Drawing for the job (mm, zero at the part's lowest x, y, z). A direction names the side the tool comes from. Give positions to 0.01 mm unless a question says otherwise; leave off trailing zeros. Order: outer loops, then holes, each group sorted by start corner. A loop starts at its lowest first (then second) coordinate and runs counter-clockwise, first axis right, second up. Notation, with made-up numbers: M 14.25,-32.5 L 50.25,-32.5 A10 ccw 50.25,-26.5 Z; hole C 0.5,72 d1. An arc over 180 degrees is marked long. Answer as a JSON object with one key per item and string values.
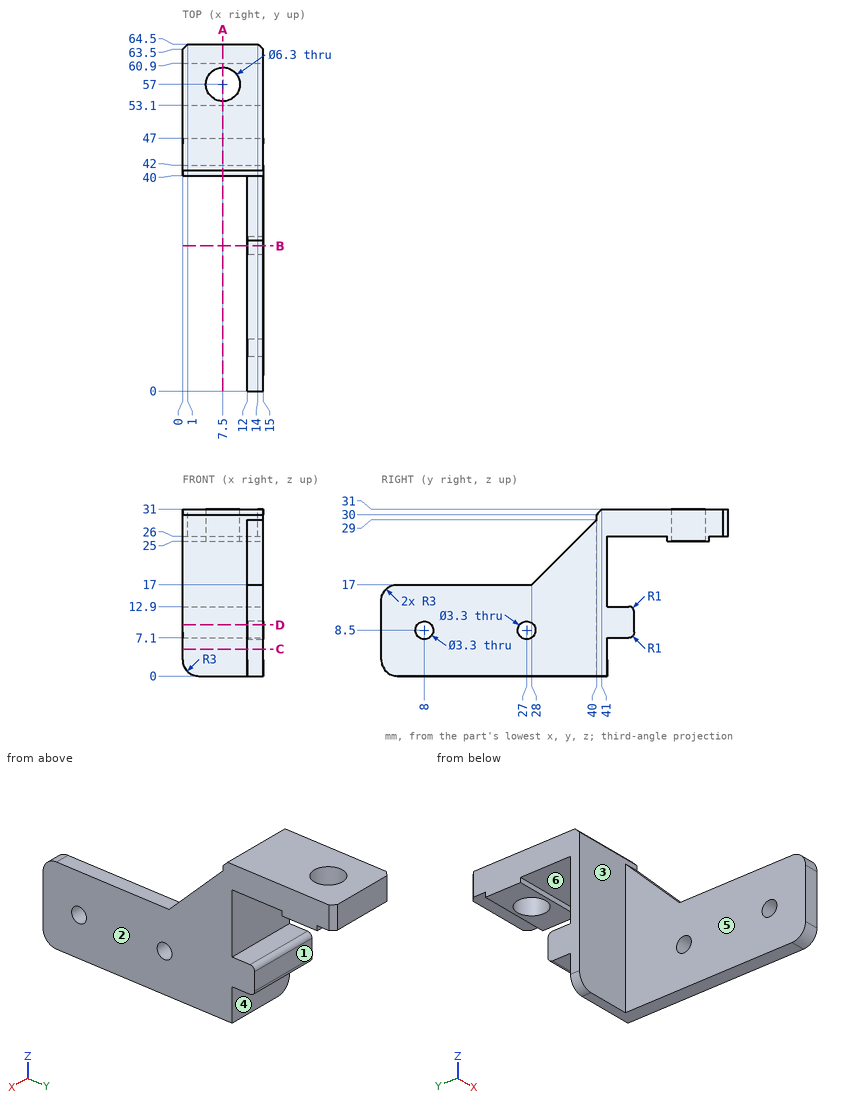
1. Pin check, flat tips, straight feed: P1, Ø5.5, axis at x = 9, y = 45.5, coming from the -Z side; P2, Ø4, axis at x = 11, z = 20.5, coming from the +Y side; P3, Ø4, axis at x = 9.5, z = 9.5, coming from the +Y side; P4, Ø2, axis at y = 27, z = 8.5, coming from the -X side. Stop position of each tip, or through.
Worked answers:
{"P1": "stops at z = 7.1", "P2": "stops at y = 42", "P3": "stops at y = 47", "P4": "passes through"}
2. Cut at A-A on x = 7.5. Give the cut face in (y, z).
Worked answers:
{"outline": "M 40,0 L 42,0 L 42,7.1 L 46,7.1 A1 ccw 47,8.1 L 47,11.9 A1 ccw 46,12.9 L 42,12.9 L 42,26 L 53.1,26 L 53.1,25 L 53.85,25 L 53.85,31 L 41,31 L 40,30 Z; M 60.15,25 L 60.9,25 L 60.9,26 L 64.5,26 L 64.5,31 L 60.15,31 Z"}
3. Cut at D-D on z = 9.5. Give the cut face in (x, y).
Worked answers:
{"outline": "M 0,40 L 12,40 L 12,28.31 L 15,28.31 L 15,47 L 0,47 Z; M 12,0 L 15,0 L 15,6.69 L 12,6.69 Z; M 12,9.31 L 15,9.31 L 15,25.69 L 12,25.69 Z"}
4. Two-plate mould, pull along Y, no slides. Class the marked faces 3, 4, 5 and 6: +Y half, -Y half, draft (parallel to the pull), parting line (faces both ways), or undercut.
Worked answers:
{"face 3": "-Y half", "face 4": "+Y half", "face 5": "draft", "face 6": "undercut"}
5. Cut at B-B on y = 27. Give the cut face in (x, z), plus the area to 3 significant figures.
Worked answers:
{"outline": "M 12,0 L 15,0 L 15,6.85 L 12,6.85 Z; M 12,10.15 L 15,10.15 L 15,17 L 12,17 Z", "area": "41.1 mm^2"}
6. Which spindle directions (+Z, -Z, +X, -X, +Y, -Y) get a long thin tool onto all of the face, cutting with end or side? Do the marked faces 1 and 2. Say none if no direction does.
Worked answers:
{"face 1": "-Z, +X, -X, +Y", "face 2": "+Z, -Z, +X, +Y, -Y"}
7. Cut at C-C on z = 5. Give the cut face in (x, y), plus the area to 3 significant figures.
Worked answers:
{"outline": "M 0,40 L 12,40 L 12,0 L 15,0 L 15,42 L 0,42 Z", "area": "150 mm^2"}
8. Probe line 1 along Y through (x, z) = (13.85, 8.5); line 2 along Z through (x, y) = (12.65, 8); line 3 along Y through (x, z) = (7.5, 26.75). List the from-to ranges inside material, lowest first.
Worked answers:
{"line 1": "y = 0 to 6.35, 9.65 to 25.35, 28.65 to 47", "line 2": "z = 0 to 6.85, 10.15 to 17", "line 3": "y = 40 to 53.85, 60.15 to 64.5"}
